Check sheet for the modelled part. Datum: model origin and axes. Units: mm. Face numbers are marked on the shaded views. Round coordinates to 2 decimals unless told otherwise and drop trailing zeros. Write each loop counter-clockwise with the first axis right and the second up, starting at its lowest first coordinate (ties: lowest second). Pieces come first, ordered by that corner, then holes.
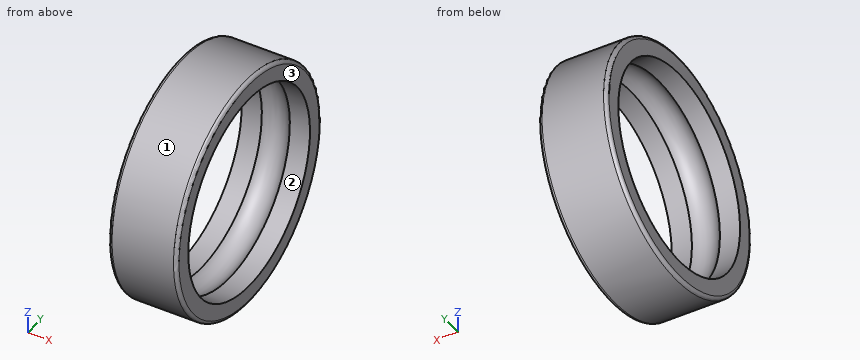
from build123d import *


with BuildPart() as part:
    # Esquisse1 → Base-R_volution (revolve)
    with BuildSketch(Plane(origin=(0, 0, 0), x_dir=(1, 0, 0), z_dir=(0, 1, 0)), mode=Mode.PRIVATE) as base_r_volution_sk:
        with BuildLine():
            Line((0, 20.4), (0, 17.7))
            Line((0, 17.7), (3.540325225, 17.7))
            ThreePointArc((3.540325225, 17.7), (6, 18.8), (8.459674775, 17.7))
            Line((8.459674775, 17.7), (12, 17.7))
            Line((12, 17.7), (12, 20.4))
            ThreePointArc((12, 20.4), (11.824264069, 20.824264069), (11.4, 21))
            Line((11.4, 21), (0.6, 21))
            ThreePointArc((0.6, 21), (0.175735931, 20.824264069), (0, 20.4))
        make_face()
    revolve(base_r_volution_sk.sketch.rotate(Axis((0, 0, 0), (1, 0, 0)), 180), axis=Axis((0, 0, 0), (1, 0, 0)))


solid = part.part
1. Sectioned sample at D-D, the plane x = 7. Enter the section's corners in (y, z), plus the area to 3 significant figures.
2. Release check for a two-part mould opening along Z. For the marked faces 1, 2 and 3 record: released by +Z, released by -Z, zero draft, split by the parting line, or undercut.
3. Sectioned sample at C-C, the plane x = 4.25. Enter the section's corners in (y, z).
4. Scan lines: line 1 along Y through (x, z) = (2.1, 0); line 2 along Z through (x, y) = (10, -12); line 3 along Z through (x, y) = (9.75, 2.5). Record each from-to range of solid material in increasing order.
5. Go/stop test with flat-tipped pins: pin 1 (6 mm diameter, centred on x = 9, y = 15, fed in from +Z); pin 2 (3 mm diameter, centred on x = 9, z = 10.5, fed in from -Y); pin 3 (4 mm diameter, centred on x = 8, y = -9, fed in from +Z). Record where each tip stops, or that it passes through.
6. Sectioned sample at A-A, the plane z = 0. Enter the section's corners in (x, y).
Computed values:
1. outline: circle Ø42 at (0, 0); hole circle Ø37.29 at (0, 0)
1. area: 293 mm2
2. face 1: split by the parting line
2. face 2: undercut
2. face 3: zero draft
3. outline: circle Ø42 at (0, 0); hole circle Ø36.6 at (0, 0)
4. line 1: y = -21 to -17.7, 17.7 to 21
4. line 2: z = -17.23 to -13.01, 13.01 to 17.23
4. line 3: z = -20.85 to -17.52, 17.52 to 20.85
5. pin 1: stops at z = 17.23
5. pin 2: stops at y = -18.97
5. pin 3: stops at z = 19.8
6. outline: (0, -20.4) arc R0.6 ccw to (0.6, -21) - (11.4, -21) arc R0.6 ccw to (12, -20.4) - (12, -17.7) - (8.46, -17.7) arc R3.3 cw to (3.54, -17.7) - (0, -17.7) - close; (0, 17.7) - (3.54, 17.7) arc R3.3 cw to (8.46, 17.7) - (12, 17.7) - (12, 20.4) arc R0.6 ccw to (11.4, 21) - (0.6, 21) arc R0.6 ccw to (0, 20.4) - close
